Work out the finished part from the listing and answer in its coordinate system (mm). A direction names the side the tool comes from. Give positions to 0.01 mm unless a question says otherwise; leave off trailing zeros. Order: outer loops, then holes, each group sorted by start corner. A loop starts at its lowest first (then second) coordinate and runs counter-clockwise, first axis right, second up.
```python
from build123d import *

# Parameters (mm, degrees)
F1_DEPTH = 30.4
F2_W     = 6.8
F2_H     = 6.8
F3_DEPTH = 50
F4_R     = 6.2
F4_R_2   = 5.5
F5_DEPTH = 4.3
F6_DEPTH = 4.3
F7_DEPTH = 2


# Not quite as in the source:
# - a feature names something its author has since deleted; it is built from what else it names


with BuildPart() as f1:
    # F0 (on Top) → F1 (new body)
    with BuildSketch(Plane.XY):
        with BuildLine():
            ThreePointArc((0, -10), (-10, 0), (0, 10))
            Line((0, 10), (-27.8, 10))
            Line((-27.8, 10), (-27.8, -10))
            Line((-27.8, -10), (0, -10))
        make_face()
        with BuildLine():
            ThreePointArc((0, -10), (7.0710678119, -7.0710678119), (10, 0))
            ThreePointArc((10, 0), (7.0710678119, 7.0710678119), (0, 10))
            Line((0, 10), (0, 6.2))
            ThreePointArc((0, 6.2), (4.3840620434, 4.3840620434), (6.2, 0))
            ThreePointArc((6.2, 0), (4.3840620434, -4.3840620434), (0, -6.2))
            Line((0, -6.2), (0, -10))
        make_face()
        with BuildLine():
            Line((0, 6.2), (0, 10))
            ThreePointArc((0, 10), (-10, 0), (0, -10))
            Line((0, -10), (0, -6.2))
            ThreePointArc((0, -6.2), (-6.2, 0), (0, 6.2))
        make_face()
        with BuildLine():
            Line((0, 5.5), (0, 6.2))
            ThreePointArc((0, 6.2), (-6.2, 0), (0, -6.2))
            Line((0, -6.2), (0, -5.5))
            ThreePointArc((0, -5.5), (-5.5, 0), (0, 5.5))
        make_face()
        with BuildLine():
            ThreePointArc((6.2, 0), (4.3840620434, 4.3840620434), (0, 6.2))
            Line((0, 6.2), (0, 5.5))
            ThreePointArc((0, 5.5), (3.8890872965, 3.8890872965), (5.5, 0))
            ThreePointArc((5.5, 0), (3.8890872965, -3.8890872965), (0, -5.5))
            Line((0, -5.5), (0, -6.2))
            ThreePointArc((0, -6.2), (4.3840620434, -4.3840620434), (6.2, 0))
        make_face()
    extrude(amount=F1_DEPTH)

    # F2 (on face) → F3 (cut)
    with BuildSketch(Plane.XZ.offset(10)):
        with Locations((-22.4, 25)):
            Rectangle(F2_W, F2_H)
        with Locations((-22.4, 5.4)):
            Rectangle(F2_W, F2_H)
    extrude(amount=-F3_DEPTH, mode=Mode.SUBTRACT)

    # F4 (on face) → F5 (cut)
    with BuildSketch(Plane.XY.offset(30.4)):
        Circle(F4_R)
        Circle(F4_R_2, mode=Mode.SUBTRACT)
    extrude(amount=-F5_DEPTH, mode=Mode.SUBTRACT)

    # F0 (on Top) → F6 (cut)
    with BuildSketch(Plane.XY):
        with BuildLine():
            ThreePointArc((6.2, 0), (4.3840620434, 4.3840620434), (0, 6.2))
            Line((0, 6.2), (0, 5.5))
            ThreePointArc((0, 5.5), (3.8890872965, 3.8890872965), (5.5, 0))
            ThreePointArc((5.5, 0), (3.8890872965, -3.8890872965), (0, -5.5))
            Line((0, -5.5), (0, -6.2))
            ThreePointArc((0, -6.2), (4.3840620434, -4.3840620434), (6.2, 0))
        make_face()
        with BuildLine():
            Line((0, 5.5), (0, 6.2))
            ThreePointArc((0, 6.2), (-6.2, 0), (0, -6.2))
            Line((0, -6.2), (0, -5.5))
            ThreePointArc((0, -5.5), (-5.5, 0), (0, 5.5))
        make_face()
    extrude(amount=F6_DEPTH, mode=Mode.SUBTRACT)

    # F2 (on face) → F7 (join)
    with BuildSketch(Plane.XZ.offset(10)):
        with Locations((-22.4, 25)):
            Rectangle(F2_W, F2_H)
        with Locations((-22.4, 5.4)):
            Rectangle(F2_W, F2_H)
    extrude(amount=-F7_DEPTH)


solid = f1.part
```
1. The part is cut by section C-C (y = -7.25). Write down the section's boundary in (x, z).
Findings below:
outline: (-27.8, 0) - (6.89, 0) - (6.89, 30.4) - (-27.8, 30.4) - close; hole (-25.8, 2) - (-19, 2) - (-19, 8.8) - (-25.8, 8.8) - close; hole (-25.8, 21.6) - (-19, 21.6) - (-19, 28.4) - (-25.8, 28.4) - close
2. The part is cut by section D-D (y = 1.75). Write down the section's boundary in (x, z), then the cut area to 3 significant figures.
Findings below:
outline: (-27.8, 0) - (-5.95, 0) - (-5.95, 4.3) - (-5.21, 4.3) - (-5.21, 26.1) - (-5.95, 26.1) - (-5.95, 30.4) - (-27.8, 30.4) - close; (5.21, 4.3) - (5.95, 4.3) - (5.95, 0) - (9.85, 0) - (9.85, 30.4) - (5.95, 30.4) - (5.95, 26.1) - (5.21, 26.1) - close; hole (-25.8, 2) - (-19, 2) - (-19, 8.8) - (-25.8, 8.8) - close; hole (-25.8, 21.6) - (-19, 21.6) - (-19, 28.4) - (-25.8, 28.4) - close
area: 722 mm2
3. Which of the six approach directions +Z, -Z, +X, -X, +Y, -Y give full straight-line access (tool end or side, diameter ignored) to faces 1 (the face through (2.86, -5.5, 28.28)), 2 (the face through (-27.8, 0, 15)), 3 (the face through (-22, 1, 8.8))?
Findings below:
face 1: +Z
face 2: +Z, -Z, -X, +Y, -Y
face 3: +Y
4. The part is cut by section A-A (y = 4.75). Write down the section's boundary in (x, z), then the cut area to 3 significant figures.
Findings below:
outline: (-27.8, 0) - (-3.98, 0) - (-3.98, 4.3) - (-2.77, 4.3) - (-2.77, 26.1) - (-3.98, 26.1) - (-3.98, 30.4) - (-27.8, 30.4) - close; (2.77, 4.3) - (3.98, 4.3) - (3.98, 0) - (8.8, 0) - (8.8, 30.4) - (3.98, 30.4) - (3.98, 26.1) - (2.77, 26.1) - close; hole (-25.8, 2) - (-19, 2) - (-19, 8.8) - (-25.8, 8.8) - close; hole (-25.8, 21.6) - (-19, 21.6) - (-19, 28.4) - (-25.8, 28.4) - close
area: 831 mm2
5. Given P1, Ø2, axis at y = 1.5, z = 6, coming from the +X side; P2, Ø2, axis at x = 3, z = 25, coming from the -Y side; P3, Ø6, axis at x = -1, y = 1.5, coming from the +Z side; P4, Ø1.5, axis at y = 3, z = 13.5, coming from the +X side, each flat-ended and moving along its own axis, determine where each tip first touches the part or whether it passes through.
Findings below:
P1: stops at x = 9.99
P2: stops at y = -9.8
P3: passes through
P4: stops at x = 9.74
6. The mould has two halves that part along Y. Classify faces 4 (the face through (-4, -4, 4.3)), 5 (the face through (-25.8, 1, 25)), 6 (the face through (-22, -8, 25)), 7 (the face through (-4, -4, 26.1)): pulls with the +Y half, pulls with the -Y half, needs draft (parallel to the pull), parting line crosses it, or undercut.
Findings below:
face 4: undercut
face 5: needs draft
face 6: pulls with the +Y half
face 7: undercut
7. Straight lines are drawn through the part: probe 1 along Z at (x, y) = (-25, -6.5); probe 2 along X at (y, z) = (5, 7); probe 3 along Y at (x, z) = (0, 28.8). For each, find the intervals that lie inside material, in ascending order.
Findings below:
probe 1: z = 0 to 2, 8.8 to 21.6, 28.4 to 30.4
probe 2: x = -27.8 to -25.8, -19 to -2.29, 2.29 to 8.66
probe 3: y = -10 to -6.2, 6.2 to 10
8. The part is cut by section B-B (z = 27.5). Write down the section's boundary in (x, y), then the cut area to 3 significant figures.
Findings below:
outline: (-27.8, -10) - (0, -10) arc R10 ccw to (0, 10) - (-19, 10) - (-19, -8) - (-25.8, -8) - (-25.8, 10) - (-27.8, 10) - close; hole circle Ø12.4 at (0, 0)
area: 470 mm2
